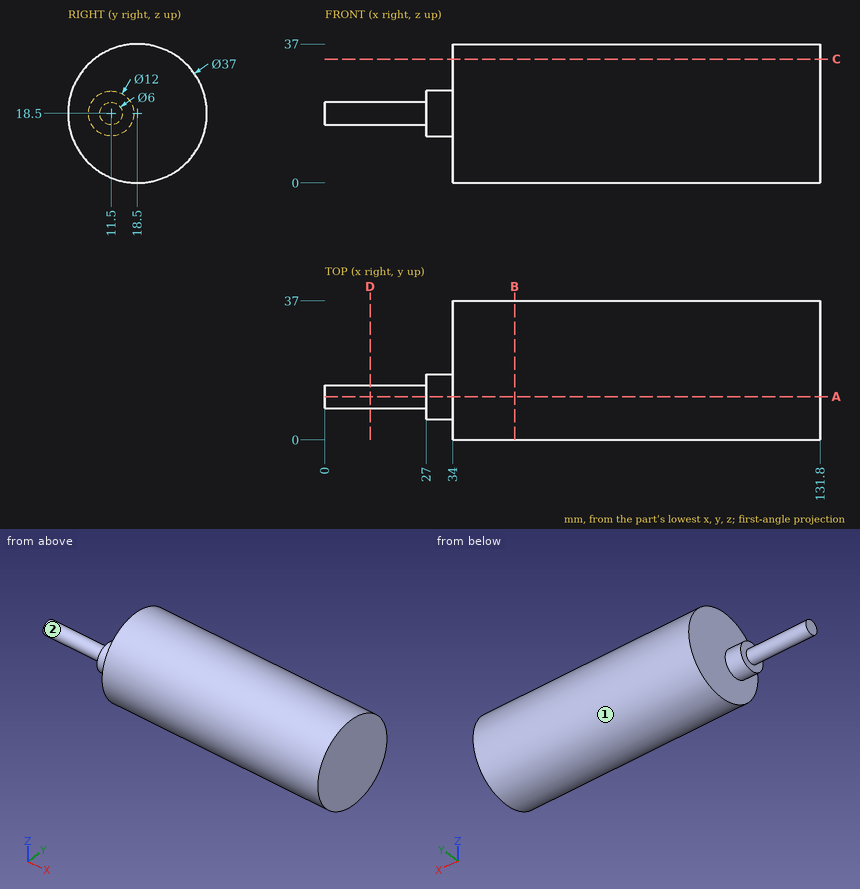
Here's the drawing with two shaded views (mm, measured from the low corner). I have some questions. A direction names the side the tool comes from. Give positions to 0.01 mm unless a question says otherwise; leave off trailing zeros. Order: outer loops, then holes, each group sorted by start corner. A loop starts at its lowest first (then second) coordinate and runs counter-clockwise, first axis right, second up. Notation, with made-up numbers: (39.5, 43.25) -> (79.5, 43.25) arc R24 ccw to (79.5, 68.25) -> close; hole circle Ø7 at (69.25, 27.25). An arc over 180 degrees is marked (long way). Use a Markdown table: item, result. Add a question column.
Item 1: Imagine slicing it at A-A on y = 11.5. Please give me the cut outline in (x, z), plus the area to 3 significant figures.
Item 2: I need wall thicknesses on line 1 (X direction, y = 20.5, z = 3.5); line 2 (X direction, y = 8, z = 14); line 3 (Z direction, x = 115, y = 19). Which ranges of each line are inside material? Lowest first, please.
Item 3: Imagine slicing it at C-C on z = 33. Please give me the cut outline in (x, y), plus the area to 3 significant figures.
Item 4: Will these pins go through, and if not, where does the flat tip stop? pin 1 (5 mm diameter, centred on x = 110, z = 13, fed in from -Y); pin 2 (1 mm diameter, centred on x = 53.5, z = 16.5, fed in from +Y); pin 3 (1 mm diameter, centred on x = 100.5, z = 8, fed in from -Y).
Item 5: Imagine slicing it at D-D on x = 12. Please give me the cut outline in (y, z), plus the area to 3 significant figures.
Item 6: For the marked faces 1 and 2, which set-ups out of +Z, -Z, +X, -X, +Y, -Y let a thin tool reach every point of the face, with its end or its side?
Item 7: Imagine slicing it at B-B on x = 50.5. Please give me the cut outline in (y, z).
Data:
| question | item | result |
|---|---|---|
| 1 | outline | (0, 15.5) -> (27, 15.5) -> (27, 12.5) -> (34, 12.5) -> (34, 1.38) -> (131.8, 1.38) -> (131.8, 35.62) -> (34, 35.62) -> (34, 24.5) -> (27, 24.5) -> (27, 21.5) -> (0, 21.5) -> close |
| 1 | area | 3,600 mm² |
| 2 | line 1 | x = 34 to 131.8 |
| 2 | line 2 | x = 27 to 131.8 |
| 2 | line 3 | z = 0.01 to 36.99 |
| 3 | outline | (34, 7.01) -> (131.8, 7.01) -> (131.8, 29.99) -> (34, 29.99) -> close |
| 3 | area | 2,250 mm² |
| 4 | pin 1 | stops at y = 0.24 |
| 4 | pin 2 | stops at y = 36.94 |
| 4 | pin 3 | stops at y = 2.94 |
| 5 | outline | circle Ø6 at (11.5, 18.5) |
| 5 | area | 28.3 mm² |
| 6 | face 1 | +X, -X |
| 6 | face 2 | -X |
| 7 | outline | circle Ø37 at (18.5, 18.5) |
